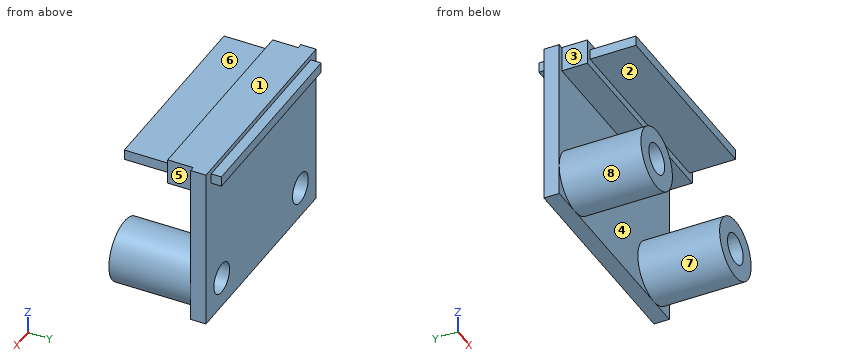
```python
from build123d import *

# Parameters (mm, degrees)
SKETCH_1_W      = 21
SKETCH_1_H      = 16
SKETCH_1_R      = 1.5
EXTRUDE_2_DEPTH = 1.5
SKETCH_1_4_W    = 19
SKETCH_1_4_H    = 1
EXTRUDE_3_DEPTH = 1
SKETCH_3_W      = 19
SKETCH_3_H      = 1
EXTRUDE_4_DEPTH = 7
SKETCH_3_3_W    = 20
SKETCH_3_3_H    = 2.5
EXTRUDE_5_DEPTH = 2.5
SKETCH_4_R      = 3
SKETCH_4_R_2    = 1.5
EXTRUDE_6_DEPTH = 8


with BuildPart() as part:
    # Sketch 1 → Extrude 2 (new body)
    with BuildSketch(Plane(origin=(0, 0, 0), x_dir=(1, 0, 0), z_dir=(0, 1, 0))):
        Rectangle(SKETCH_1_W, SKETCH_1_H)
        with Locations(Location((-7.5, 5, 0), (0, 0, 270))):
            Circle(SKETCH_1_R, mode=Mode.SUBTRACT)
        with Locations(Location((7.5, 5, 0), (0, 0, 270))):
            Circle(SKETCH_1_R, mode=Mode.SUBTRACT)
    extrude(amount=-EXTRUDE_2_DEPTH)

    # Sketch 1_4 → Extrude 3 (add)
    with BuildSketch(Plane(origin=(0, 0, 0), x_dir=(1, 0, 0), z_dir=(0, 1, 0))):
        with Locations((0, -7)):
            Rectangle(SKETCH_1_4_W, SKETCH_1_4_H)
    extrude(amount=EXTRUDE_3_DEPTH)

    # Sketch 3 → Extrude 4 (add)
    with BuildSketch(Plane.XZ.offset(1.5)):
        with Locations((0, 6.75)):
            Rectangle(SKETCH_3_W, SKETCH_3_H)
    extrude(amount=EXTRUDE_4_DEPTH)

    # Sketch 3_3 → Extrude 5 (add)
    with BuildSketch(Plane.XZ.offset(1.5)):
        with Locations((0, 6.75)):
            Rectangle(SKETCH_3_3_W, SKETCH_3_3_H)
    extrude(amount=EXTRUDE_5_DEPTH)

    # Sketch 4 → Extrude 6 (add)
    # profile 1 of 2: a face of its own
    with BuildSketch(Plane.XZ.offset(1.5)):
        with Locations(Location((-7.5, -5, 0), (0, 0, 270))):
            Circle(SKETCH_4_R)
        with Locations(Location((-7.5, -5, 0), (0, 0, 90))):
            Circle(SKETCH_4_R_2, mode=Mode.SUBTRACT)
    # profile 2 of 2: a face of its own
    with BuildSketch(Plane.XZ.offset(1.5)):
        with Locations(Location((7.5, -5, 0), (0, 0, 270))):
            Circle(SKETCH_4_R)
        with Locations(Location((7.5, -5, 0), (0, 0, 90))):
            Circle(SKETCH_4_R_2, mode=Mode.SUBTRACT)
    extrude(amount=EXTRUDE_6_DEPTH)


solid = part.part
```
Check sheet for the modelled part. Datum: model origin and axes. Units: mm. Face numbers are marked on the shaded views. A direction names the side the tool comes from. Give positions to 0.01 mm unless a question says otherwise; leave off trailing zeros. Loops run counter-clockwise (first coordinate to the right, second up) from the corner with the lowest first, then second, coordinate; pieces in that order, holes last. Notation, with made-up numbers: (-12.5, -17.5) - (45.5, -17.5) arc R37 cw to (45.5, 20.5) - close; hole circle Ø10 at (78.5, 35). An arc over 180 degrees is marked (long way). One line per question, with ' | ' between items. Start each with the question number.
1. Gauge pin test, flat ends, axial feed: pin 1 Ø3.5 at (x, z) = (7.5, -5) entering from +Y; pin 2 Ø4 at (x, z) = (3, 2) entering from -Y; pin 3 Ø2 at (x, y) = (4.5, -7) entering from -Z. Record the tip position at first contact, or that the pin passes through.
2. Cross-section at B-B, the plane x = -3.75. Enter the section's corners in (y, z).
3. Cross-section at C-C, the plane x = 8. Enter the section's corners in (y, z).
4. Draft check along Z on the marked faces 5, 6, 7 and 8. Enter one of: released by +Z, released by -Z, zero draft, split by the parting line, or undercut.
5. Cross-section at D-D, the plane z = 4.5. Enter the section's corners in (x, y), plus the area to 3 significant figures.
6. Material ranges on line 1 along X through (y, z) = (-0.6, -5); line 2 along X through (y, z) = (-6.25, -5); line 3 along X through (y, z) = (-2.75, -4), recorded low to high. Write a range as [from, to].
7. Cross-section at A-A, the plane y = -3.75. Enter the section's corners in (x, z).
8. Set-up check for the marked faces 1, 2, 3 and 4: record each of +Z, -Z, +X, -X, +Y, -Y from which the full face is reachable in a straight line by a thin tool's end or side.
Check result:
1) pin 1: stops at y = 0 | pin 2: stops at y = -1.5 | pin 3: stops at z = -7.24
2) outline: (-8.5, 6.25) - (-4, 6.25) - (-4, 5.5) - (-1.5, 5.5) - (-1.5, -8) - (0, -8) - (0, 6.5) - (1, 6.5) - (1, 7.5) - (0, 7.5) - (0, 8) - (-4, 8) - (-4, 7.25) - (-8.5, 7.25) - close
3) outline: (-9.5, -7.96) - (-1.5, -7.96) - (-1.5, -8) - (0, -8) - (0, -6.41) - (-9.5, -6.41) - close; (-9.5, -3.59) - (0, -3.59) - (0, 6.5) - (1, 6.5) - (1, 7.5) - (0, 7.5) - (0, 8) - (-4, 8) - (-4, 7.25) - (-8.5, 7.25) - (-8.5, 6.25) - (-4, 6.25) - (-4, 5.5) - (-1.5, 5.5) - (-1.5, -2.04) - (-9.5, -2.04) - close
4) face 5: zero draft | face 6: released by +Z | face 7: undercut | face 8: undercut
5) outline: (-10.5, -1.5) - (10.5, -1.5) - (10.5, 0) - (-10.5, 0) - close | area: 31.5 mm2
6) line 1: x = [-10.5, -9], [-6, 6], [9, 10.5] | line 2: x = [-10.5, -9], [-6, -4.5], [4.5, 6], [9, 10.5] | line 3: x = [-10.33, -8.62], [-6.38, -4.67], [4.67, 6.38], [8.62, 10.33]
7) outline: circle Ø6 at (-7.5, -5); (-10, 5.5) - (10, 5.5) - (10, 8) - (-10, 8) - close; circle Ø6 at (7.5, -5); hole circle Ø3 at (-7.5, -5); hole circle Ø3 at (7.5, -5)
8) face 1: +Z, +X, -X, +Y, -Y | face 2: +X, -X, -Y | face 3: +Z, -X, -Y | face 4: -Y
